Input: part model. Units: mm. Frame: model coordinates. A direction names the side the tool comes from. Round coordinates to 2 decimals unless told otherwise and drop trailing zeros. Order: outer loops, then holes, each group sorted by start corner. A loop starts at its lowest first (then second) coordinate and runs counter-clockwise, first axis right, second up. Notation, with made-up numbers: (42.5, 3.5) -> (85.5, 3.5) arc R19 ccw to (85.5, 18.5) -> close; hole circle Ø3 at (3.25, 53). An arc over 180 degrees is marked (long way). Use a Markdown table: item, result.
Autodesk Inventor part; units mm, degrees
ref_plane "Work Plane1" through (0, 0, 0) normal (0, 0, 1) x (1, 0, 0)
ref_plane "Work Plane2" through (-18.2218, -48.2782, 35.3062) normal (0, 0, 1) x (1, 0, 0)
ref_plane "Work Plane3" through (0, 0, 5) normal (0, 0, -1) x (-1, 0, 0)
ref_plane "Work Plane1" through (0, 0, 0) normal (0, 0, 1) x (1, 0, 0)
sketch "Sketch1" plane through (0, 0, 0) normal (0, 0, 1) x (1, 0, 0)
  circle A0 centre (1.7782, -8.2782) radius 7.5245 construction
  line L0 (-2.7782, -19.2782) -> (-13.7782, -8.2782) construction
  line L1 (13.7782, -19.2782) -> (-2.7782, -19.2782) construction
  line L2 (13.7782, 19.2782) -> (13.7782, -19.2782) construction
  line L3 (-13.7782, -8.2782) -> (13.7782, 19.2782) construction
  line L4 (13.8782, -19.2782) -> (-2.7782, -19.2782)
  line L5 (-2.7782, -19.2782) -> (-13.2782, -8.7782)
  circle A1 centre (1.7782, -8.2782) radius 7.5245
  line L6 (-13.2782, -7.7782) -> (12.8782, 18.3782)
  line L7 (-13.7782, -8.2782) -> (13.7782, 19.2782) construction
  line L8 (13.7782, 19.2782) -> (13.7782, 36.7218) construction
  line L9 (13.7782, 36.7218) -> (-18.2218, 36.7218) construction
  line L10 (-13.2782, -7.7782) -> (-13.2782, -8.7782)
  line L11 (20.8782, 32.7218) -> (13.8782, 32.7218)
  line L12 (13.8782, -33.6218) -> (20.8782, -33.6218)
  line L13 (20.8782, -33.6218) -> (20.8782, 32.7218)
  line L14 (13.8782, 18.3782) -> (12.8782, 18.3782)
  line L15 (13.8782, 32.7218) -> (13.8782, 18.3782)
  line L16 (13.8782, -19.2782) -> (13.8782, -33.6218)
  line L17 (13.7782, -19.2782) -> (-2.7782, -19.2782)
  line L18 (-2.7782, -19.2782) -> (-13.7782, -8.2782)
  line L19 (-18.2218, 36.7218) -> (-18.2218, -48.2782)
  line L20 (-18.2218, -48.2782) -> (13.7782, -48.2782)
  line L21 (13.7782, -48.2782) -> (13.7782, -19.2782)
  point P0 (0, 0)
  dimension "d0" = 0
  dimension "d4" = 0.1
  dimension "d5" = 1
  dimension "d6" = 1
  dimension "d7" = 0
  dimension "d8" = 0
  dimension "d9" = 0
  dimension "d10" = 7
  dimension "d11" = 4
  dimension "d13" = 66.3436
ref_plane "Work Plane2" through (-18.2218, -48.2782, 35.3062) normal (0, 0, 1) x (1, 0, 0)
extrude "Main Part Body" add sketch "Sketch1" along normal blind 35
ref_plane "Work Plane3" through (0, 0, 5) normal (0, 0, -1) x (-1, 0, 0)
sketch "Sketch2" plane through (-2.7782, -19.2782, 35) normal (0, 0, 1) x (1, 0, 0)
  circle A0 centre (4.5563, 11) radius 9
  circle A1 centre (4.5563, 11) radius 7.5245 construction
  dimension "d59" = 18
extrude "Bore for SM05" cut sketch "Sketch2" against normal up to surface (30 mm away)
sketch "Sketch3" plane through (20.8782, -33.6218, 35.3062) normal (1, 0, 0) x (0, 0, -1)
  circle A0 centre (22.3062, 25.3437) radius 2.3
  circle A1 centre (8.3062, 25.3437) radius 2.3
  line L0 (42.3062, 25.3437) -> (-6.6938, 25.3437) construction
  line L1 (30.3062, 79.6124) -> (30.3062, -13.2687) construction
  line L2 (35.3062, 0) -> (35.3062, 66.3437) construction
  line L3 (35.3062, 66.3437) -> (0.3062, 66.3437) construction
  line L4 (0.3062, 0) -> (0.3062, 66.3437) construction
  line L5 (35.3062, 0) -> (0.3062, 0) construction
  point P0 (35.3062, 33.6218)
  dimension "d21" = 4.6
  dimension "d22" = 4.6
  dimension "d27" = 8
  dimension "d52" = 8
extrude "Thru Holes for Lens Tube Set Screws M4" cut sketch "Sketch3" against normal up to next
sketch "Sketch4" plane through (20.8782, -33.6218, 0) normal (1, 0, 0) x (0, 0, -1)
  circle A0 centre (-13, 25.3437) radius 2.3 construction
  circle A1 centre (-27, 25.3437) radius 2.3 construction
  point P0 (0, 33.6218)
hole "Holes for Set Screw Insert M4" at (20.8782, -8.2782, 13) at (20.8782, -8.2782, 27) direction (-1, 0, 0) diameter 5.6 depth 9.1
sketch "Sketch6" plane through (0, 0, 0) normal (0, 0, -1) x (-1, 0, 0)
  line L0 (-20.8782, -33.6218) -> (-20.8782, 32.7218) construction
  line L1 (-13.8782, -33.6218) -> (-20.8782, -33.6218) construction
  line L2 (-13.8782, -19.2782) -> (-13.8782, -33.6218) construction
  line L3 (2.7782, -19.2782) -> (-13.8782, -19.2782) construction
  line L4 (13.2782, -8.7782) -> (2.7782, -19.2782) construction
  line L5 (13.2782, -7.7782) -> (13.2782, -8.7782) construction
  line L6 (-12.8782, 18.3782) -> (13.2782, -7.7782) construction
  line L7 (-13.8782, 18.3782) -> (-12.8782, 18.3782) construction
  line L8 (-13.8782, 32.7218) -> (-13.8782, 18.3782) construction
  line L9 (-20.8782, 32.7218) -> (-13.8782, 32.7218) construction
  circle A0 centre (-1.7782, -8.2782) radius 7.5245 construction
  line L10 (-20.8782, 32.7218) -> (-13.8782, 32.7218)
  line L11 (-13.8782, 32.7218) -> (-13.8782, -33.6218)
  line L12 (-13.8782, -33.6218) -> (-20.8782, -33.6218)
  line L13 (-20.8782, -33.6218) -> (-20.8782, 32.7218)
  point P0 (0, 0)
extrude "Extrusion5" cut sketch "Sketch6" against normal blind 5
sketch "Sketch5" plane through (20.8782, -33.6218, 0) normal (1, 0, 0) x (0, 0, -1)
  circle A0 centre (-27, 25.3437) radius 2.8 construction
  circle A1 centre (-13, 25.3437) radius 2.8 construction
  line L0 (-5, 0) -> (-35, 0) construction
  line L1 (-5, 66.3437) -> (-35, 66.3437) construction
  line L2 (0, 52) -> (-5, 52) construction
  line L3 (0, 14.3437) -> (-5, 14.3437) construction
  line L4 (0, 33.1718) -> (-35, 33.1718) construction
  line L5 (-35.6124, 59) -> (-5, 59) construction
  line L6 (-11, 59) -> (-16, 59) construction
  line L7 (-11, 60.75) -> (-16, 60.75)
  line L8 (-16, 57.25) -> (-11, 57.25)
  arc A2 (-11, 57.25) -> (-11, 60.75) centre (-11, 59) ccw
  arc A3 (-16, 60.75) -> (-16, 57.25) centre (-16, 59) ccw
  line L9 (-24, 59) -> (-29, 59) construction
  line L10 (-24, 60.75) -> (-29, 60.75)
  line L11 (-29, 57.25) -> (-24, 57.25)
  arc A4 (-24, 57.25) -> (-24, 60.75) centre (-24, 59) ccw
  arc A5 (-29, 60.75) -> (-29, 57.25) centre (-29, 59) ccw
  line L12 (-11, 5.5937) -> (-16, 5.5937)
  line L13 (-16, 9.0937) -> (-11, 9.0937)
  arc A6 (-11, 5.5937) -> (-11, 9.0937) centre (-11, 7.3437) ccw
  arc A7 (-16, 9.0937) -> (-16, 5.5937) centre (-16, 7.3437) ccw
  line L14 (-24, 5.5937) -> (-29, 5.5937)
  line L15 (-29, 9.0937) -> (-24, 9.0937)
  arc A8 (-24, 5.5937) -> (-24, 9.0937) centre (-24, 7.3437) ccw
  arc A9 (-29, 9.0937) -> (-29, 5.5937) centre (-29, 7.3437) ccw
  line L16 (-5, 0) -> (-5, 66.3437)
  line L17 (-35, 0) -> (-35, 66.3437)
  point P0 (0, 33.6218)
  point P1 (-13.5, 59)
  point P2 (-26.5, 59)
  dimension "d37" = 7
  dimension "d40" = 5
  dimension "d41" = 5
  dimension "d42" = 3.5
  dimension "d43" = 3.5
  dimension "d51" = 8
  dimension "d54" = 6
  dimension "d55" = 6
extrude "Slots for Holddown Screws" cut sketch "Sketch5" against normal through all
equation "\"d22\" = d21"
equation "\"d52\" = d27"
equation "\"d41\" = d40"
equation "\"d43\" = d42"
properties part number "Cuvette Holder Adjustable Recv"
1) Line query: L1, parallel to Y at x = 14, z = 13; L2, parallel to Z at x = 11, y = -7; L3, parallel to Z at x = 18, y = 19. Output: solid intervals per line, ascending. Write a range as [from, to].
Results found:
| item | result |
|---|---|
| L1 | y = [-33.62, -28.03], [-24.53, -11.08], [-5.48, 23.63], [27.13, 32.72] |
| L2 | z = [0, 11.09], [14.91, 25.09], [28.91, 35] |
| L3 | z = [5, 35] |
2) Set-up query: faces 5 (the flat face through (13.878, 26, 20)), 6 (the cylindrical face through (11.138, -9.678, 14.825)), 7 (the flat face through (17, -24.528, 14)), 8 (the flat face through (6, -19.278, 17)). Return all of +Z, -Z, +X, -X, +Y, -Y with unobstructed straight access to the full face (end or side cutting, diameter ignored); none if empty.
Results found:
| item | result |
|---|---|
| face 5 | +Z, -Z, -X, +Y |
| face 6 | +X |
| face 7 | +X, -X |
| face 8 | +Z, -Z, -X, -Y |
3) Cut plane D-D on y = -14. Return loops of the section in (x, z).
Results found:
| item | result |
|---|---|
| outline | (-8.06, 0) -> (-3.11, 0) -> (-3.11, 5) -> (-5.17, 5) -> (-5.17, 35) -> (-8.06, 35) -> close; (6.66, 0) -> (13.88, 0) -> (13.88, 5) -> (20.88, 5) -> (20.88, 35) -> (8.73, 35) -> (8.73, 5) -> (6.66, 5) -> close |
4) Pin query (flat end, axial travel): pin 1 Ø16 at (y, z) = (-27, 23.5) entering from -X; pin 2 Ø5 at (y, z) = (16, 30) entering from -X; pin 3 Ø2 at (x, z) = (3.5, 29) entering from +Y. Return the tip coordinate at first contact, or that it passes through.
Results found:
| item | result |
|---|---|
| pin 1 | stops at x = -3.06 |
| pin 2 | stops at x = 8 |
| pin 3 | stops at y = 10 |
5) Pull-direction query (X, two-part tool) for faces 1 (the cylindrical face through (0.606, 0.645, 20.21)), 2 (the flat face through (20.878, -1, 20)), 3 (the flat face through (13.878, -26, 20)), 4 (the cylindrical face through (17.43, 25.34, 22.25)); classes: +X half, -X half, draft (parallel to the pull), parting line (faces both ways), or undercut.
Results found:
| item | result |
|---|---|
| face 1 | undercut |
| face 2 | +X half |
| face 3 | -X half |
| face 4 | draft |
6) Cut plane B-B on y = -26.5. Return loops of the section in (x, z), and give its area (3 significant figures).
Results found:
| item | result |
|---|---|
| outline | (13.88, 5) -> (20.88, 5) -> (20.88, 9.26) -> (13.88, 9.26) -> close; (13.88, 17.74) -> (20.88, 17.74) -> (20.88, 22.26) -> (13.88, 22.26) -> close; (13.88, 30.74) -> (20.88, 30.74) -> (20.88, 35) -> (13.88, 35) -> close |
| area | 91.4 mm² |
7) Cut plane A-A on z = 27. Return loops of the section in (x, y).
Results found:
| item | result |
|---|---|
| outline | (-13.28, -8.78) -> (-2.78, -19.28) -> (13.88, -19.28) -> (13.88, -24.53) -> (20.88, -24.53) -> (20.88, -11.08) -> (11.78, -11.08) -> (11.78, -10.58) -> (10.48, -10.58) arc R9 cw (long way) to (10.48, -5.98) -> (11.78, -5.98) -> (11.78, -5.48) -> (20.88, -5.48) -> (20.88, 23.63) -> (13.88, 23.63) -> (13.88, 18.38) -> (12.88, 18.38) -> (-13.28, -7.78) -> close; (13.88, -33.62) -> (20.88, -33.62) -> (20.88, -28.03) -> (13.88, -28.03) -> close; (13.88, 27.13) -> (20.88, 27.13) -> (20.88, 32.72) -> (13.88, 32.72) -> close |
8) Cut plane C-C on x = -0.5. Return loops of the section in (y, z), and give its area (3 significant figures).
Results found:
| item | result |
|---|---|
| outline | (-19.28, 0) -> (-15.45, 0) -> (-15.45, 5) -> (-16.99, 5) -> (-16.99, 35) -> (-19.28, 35) -> close; (-1.11, 0) -> (5, 0) -> (5, 35) -> (0.43, 35) -> (0.43, 5) -> (-1.11, 5) -> close |
| area | 256 mm² |
